Input: part model. Units: mm. Frame: model coordinates. A direction names the side the tool comes from. Coordinates: 2 decimals unless noted, no trailing zeros. Order: outer loops, then holes, each group sorted by start corner. A loop starts at its lowest first (then second) coordinate and runs counter-clockwise, first axis right, second up. Notation, with made-up numbers: (-2, -16) -> (11, -16) arc R19 cw to (11, -12) -> close; hole circle Ø2 at (11.25, 82.5). An arc over 180 degrees is marked (long way). One line per question, with ' | ' between items.
```python
from build123d import *

# Parameters (mm, degrees)
SKETCH1_W               = 30
SKETCH1_H               = 55.7
BOSS_EXTRUDE1_DEPTH     = 3
SKETCH2_W               = 4.9
SKETCH2_H               = 8
BOSS_EXTRUDE2_DEPTH     = 8
SKETCH3_R               = 1.6
CUT_EXTRUDE1_DEPTH      = 43.386583962
SKETCH4_R               = 1.5
CUT_EXTRUDE2_DEPTH      = 10
FILLET3_R               = 0.5
FILLET4_R               = 3
CUT_EXTRUDE4_DEPTH      = 33.628553446
CUT_EXTRUDE4_DEPTH_BACK = 10
FILLET5_R               = 1.5
CHAMFER1_SIZE           = 6
SKETCH6_W               = 20.2
SKETCH6_H               = 6
BOSS_EXTRUDE3_DEPTH     = 1.4


with BuildPart() as part:
    # Sketch1 → Boss-Extrude1 (new body)
    with BuildSketch(Plane.XY):
        Rectangle(SKETCH1_W, SKETCH1_H)
    extrude(amount=BOSS_EXTRUDE1_DEPTH)

    # Sketch2 → Boss-Extrude2 (add)
    with BuildSketch(Plane.XY.offset(3)):
        with Locations((-12.55, -23.85)):
            Rectangle(SKETCH2_W, SKETCH2_H)
    boss_extrude2 = extrude(amount=BOSS_EXTRUDE2_DEPTH)

    # Sketch3 → Cut-Extrude1 (cut, through all)
    with BuildSketch(Plane.ZY.offset(15)):
        with Locations((7, -23.85)):
            Circle(SKETCH3_R)
    cut_extrude1 = extrude(amount=-CUT_EXTRUDE1_DEPTH, mode=Mode.SUBTRACT)

    # Mirror1: Boss-Extrude2, Cut-Extrude1 across plane
    add(boss_extrude2.mirror(Plane(origin=(0, 0, 0), x_dir=(0, 0, 1), z_dir=(1, 0, 0))))
    add(cut_extrude1.mirror(Plane(origin=(0, 0, 0), x_dir=(0, 0, 1), z_dir=(1, 0, 0))), mode=Mode.SUBTRACT)

    # Sketch4 → Cut-Extrude2 (cut)
    with BuildSketch(Plane.XY.offset(3)):
        with Locations((0, 24.85)):
            Circle(SKETCH4_R)
    extrude(amount=-CUT_EXTRUDE2_DEPTH, mode=Mode.SUBTRACT)

    # Fillet3
    fillet3_edges = [part.edges().sort_by_distance(p)[0] for p in [
        (-1.5, 24.85, 0),
        (-1.5, 24.85, 3),
    ]]
    fillet(fillet3_edges, radius=FILLET3_R)

    # Fillet4
    fillet4_edges = [part.edges().sort_by_distance(p)[0] for p in [
        (0, -27.85, 0),
    ]]
    fillet(fillet4_edges, radius=FILLET4_R - 0.0001)  # a hair under: the kernel refuses the full size

    # Sketch5 → Cut-Extrude4 (cut, two sides: drawn at the far end of the back side and taken through both)
    with BuildSketch(Plane.XY.offset(3).offset(-CUT_EXTRUDE4_DEPTH_BACK)):
        Polygon((10.1, -27.85), (10.1, -19.85), (-10.1, -19.85), (-10.1, -27.85), (-10.1, -30.330641118), (10.1, -30.330641118), align=None)
    extrude(amount=CUT_EXTRUDE4_DEPTH + CUT_EXTRUDE4_DEPTH_BACK, mode=Mode.SUBTRACT)

    # Fillet5
    fillet5_edges = [part.edges().sort_by_distance(p)[0] for p in [
        (-12.55, -27.85, 11),
        (-12.55, -19.85, 11),
        (12.55, -19.85, 11),
        (12.55, -27.85, 11),
    ]]
    fillet(fillet5_edges, radius=FILLET5_R)

    # Chamfer1
    chamfer1_edges = [part.edges().sort_by_distance(p)[0] for p in [
        (-12.55, -19.85, 3),
        (12.55, -19.85, 3),
    ]]
    chamfer(chamfer1_edges, length=CHAMFER1_SIZE)

    # Sketch6 → Boss-Extrude3 (add)
    with BuildSketch(Plane.XY.offset(3)):
        with Locations((0, -16.85)):
            Rectangle(SKETCH6_W, SKETCH6_H)
    extrude(amount=BOSS_EXTRUDE3_DEPTH)


solid = part.part
```
1. Pin query (flat end, axial travel): pin 1 Ø9 at (x, y) = (-3.5, 4) entering from +Z; pin 2 Ø6.5 at (x, y) = (1, -17.5) entering from +Z; pin 3 Ø0.6 at (x, z) = (-11.5, 9.5) entering from +Y. Return the tip coordinate at first contact, or that it passes through.
Recorded:
pin 1: stops at z = 3 | pin 2: stops at z = 4.4 | pin 3: stops at y = -19.85
2. Ray query, line 1 (Y direction, x = 0, z = 1.75); line 2 (Z direction, x = 5.25, y = 19.5); line 3 (Y direction, x = 4, z = 3.75). Return the intervals inside material, ascending. Write a range as [from, to].
Recorded:
line 1: y = [-19.85, 23.35], [26.35, 27.85] | line 2: z = [0, 3] | line 3: y = [-19.85, -13.85]
3. Mould query, pull axis Z, two halves, no side actions, for faces 4 (the face through (15, -7, 2)), 5 (the face through (-12.58, -24.82, 5.73)), 6 (the face through (13, -24, 11)). Classes: released by +Z, released by -Z, zero draft, split by the parting line, or undercut.
Recorded:
face 4: zero draft | face 5: undercut | face 6: released by +Z
4. Cut plane B-B, the plane y = 24.85. Return loops of the section in (x, z).
Recorded:
outline: (-15, 0) -> (-2, 0) arc R0.5 ccw to (-1.5, 0.5) -> (-1.5, 2.5) arc R0.5 ccw to (-2, 3) -> (-15, 3) -> close; (1.5, 0.5) arc R0.5 ccw to (2, 0) -> (15, 0) -> (15, 3) -> (2, 3) arc R0.5 ccw to (1.5, 2.5) -> close
5. Cut plane A-A, the plane x = 0. Return loops of the section in (y, z).
Recorded:
outline: (-19.85, 0) -> (22.85, 0) arc R0.5 ccw to (23.35, 0.5) -> (23.35, 2.5) arc R0.5 ccw to (22.85, 3) -> (-13.85, 3) -> (-13.85, 4.4) -> (-19.85, 4.4) -> close; (26.35, 0.5) arc R0.5 ccw to (26.85, 0) -> (27.85, 0) -> (27.85, 3) -> (26.85, 3) arc R0.5 ccw to (26.35, 2.5) -> close
6. Cut plane C-C, the plane z = 7. Return loops of the section in (x, y), and give its area (3 significant figures).
Recorded:
outline: (-15, -27.85) -> (-10.1, -27.85) -> (-10.1, -25.45) -> (-15, -25.45) -> close; (-15, -22.25) -> (-10.1, -22.25) -> (-10.1, -17.85) -> (-15, -17.85) -> close; (10.1, -27.85) -> (15, -27.85) -> (15, -25.45) -> (10.1, -25.45) -> close; (10.1, -22.25) -> (15, -22.25) -> (15, -17.85) -> (10.1, -17.85) -> close | area: 66.6 mm^2
7. Access query for faces 1 (the face through (-12.58, -16.81, 5.96)), 2 (the face through (0, -19.85, 2)), 3 (the face through (12.58, -16.89, 6.04)). Directions: +Z, -Z, +X, -X, +Y, -Y. A direction counts if a zero-diameter tool reaches every point of the face in a straight line with its end or side. Return the directions, or none.
Recorded:
face 1: +Z, -X, +Y | face 2: +Z, -Z, -Y | face 3: +Z, +X, +Y
8. Cut plane D-D, the plane x = -12.5. Return loops of the section in (y, z).
Recorded:
outline: (-27.85, 3) arc R3 ccw to (-24.85, 0) -> (27.85, 0) -> (27.85, 3) -> (-13.85, 3) -> (-19.85, 9) -> (-19.85, 9.5) arc R1.5 ccw to (-21.35, 11) -> (-26.35, 11) arc R1.5 ccw to (-27.85, 9.5) -> close; hole circle Ø3.2 at (-23.85, 7)
